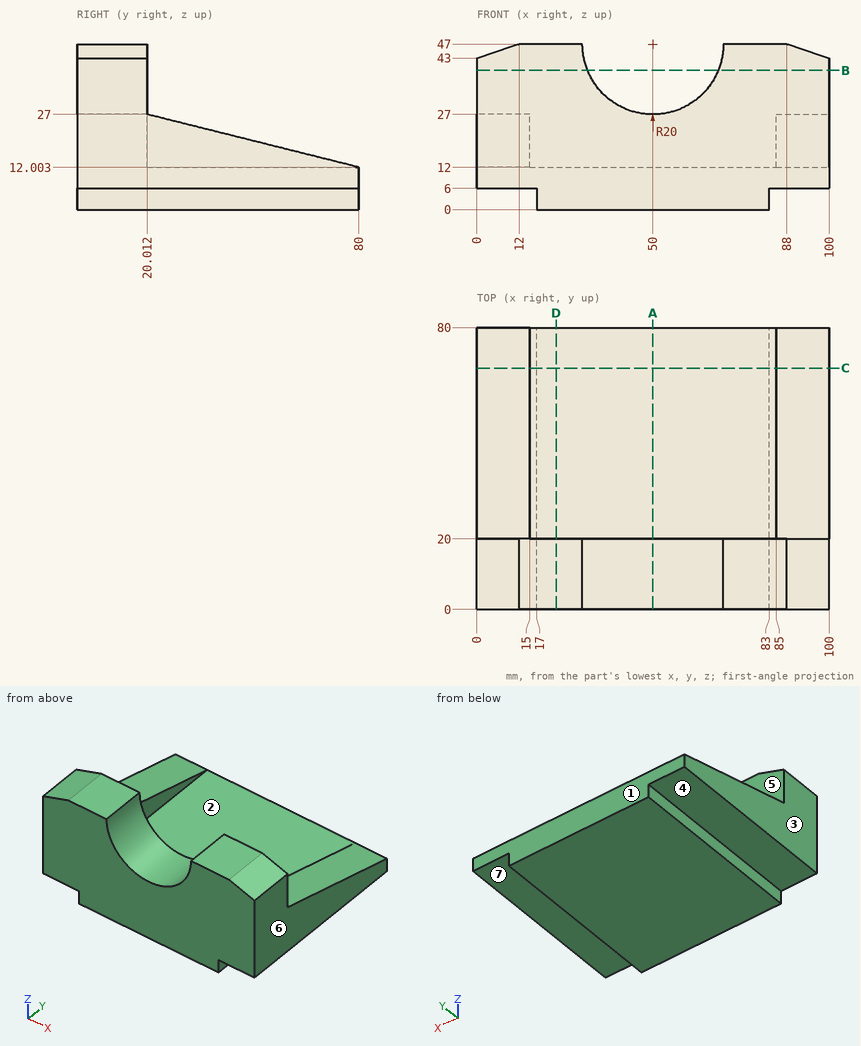
For this review, use the dimensioned drawing (mm, ordinates from the lowest corner) and the shaded views. A direction names the side the tool comes from. Give positions to 0.01 mm unless a question says otherwise; leave off trailing zeros. Write each loop counter-clockwise with the first axis right and the second up, starting at its lowest first coordinate (ties: lowest second). Pieces come first, ordered by that corner, then holes. Notation, with made-up numbers: M -8,60 L 12,60 A22 cw 12,78 Z; hole C 2,19 d9. An arc over 180 degrees is marked long. Answer as a JSON object with one key per item and string values. Group by question number.
1) We need section B-B (z = 39.5). Give the boundary of the cut face in (x, y).
2) Tool access review of the marked faces 4, 5, 6 and 7: name each direction out of +Z, -Z, +X, -X, +Y, -Y from which nothing blocks a thin tool from reaching the whole face with its end or side.
3) For line 1 along X through (y, z) = (41.5, 21); line 2 along Y through (x, z) = (34.5, 30); line 3 along Z through (x, y) = (41, 29), list the stretches that pass through material, from the lowest coordinate up.
4) We need section D-D (x = 22.5). Give the boundary of the cut face in (y, z), and give its area (3 significant figures).
5) Mouldability with a two-part tool opening along X and no side actions: class the marked faces 1, 2 and 3 as released by +X, released by -X, zero draft, split by the parting line, or undercut.
6) We need section A-A (x = 50). Give the boundary of the cut face in (y, z), and give its area (3 significant figures).
7) Clearance check with flat-ended pins moving along their axes: pin 1 Ø8 at (x, y) = (62.5, 57) entering from +Z; pin 2 Ø6.5 at (y, z) = (23, 2.5) entering from +X; pin 3 Ø1.8 at (y, z) = (58.5, 3) entering from -X. State where each tip first meets the part, or that it passes through.
8) We need section C-C (y = 68.5). Give the boundary of the cut face in (x, z), and give its area (3 significant figures).
Answer key:
{
 "1": {"outline": "M 0,0 L 31.46,0 L 31.46,20 L 0,20 Z; M 68.54,0 L 100,0 L 100,20 L 68.54,20 Z"},
 "2": {"face 4": "-Z, -X, +Y, -Y", "face 5": "+Z, +Y", "face 6": "+Z, -Z, +X, +Y, -Y", "face 7": "-Z, +X, +Y, -Y"},
 "3": {"line 1": "x = 0 to 15, 85 to 100", "line 2": "y = 0 to 20", "line 3": "z = 0 to 12"},
 "4": {"outline": "M 0,0 L 80,0 L 80,12 L 20,12 L 20,47 L 0,47 Z", "area": "1,660 mm²"},
 "5": {"face 1": "zero draft", "face 2": "undercut", "face 3": "released by -X"},
 "6": {"outline": "M 0,0 L 80,0 L 80,12 L 20,12 L 20,27 L 0,27 Z", "area": "1,260 mm²"},
 "7": {"pin 1": "stops at z = 12", "pin 2": "stops at x = 83", "pin 3": "stops at x = 17"},
 "8": {"outline": "M 0,6 L 17,6 L 17,0 L 83,0 L 83,6 L 100,6 L 100,14.88 L 85,14.88 L 85,12 L 15,12 L 15,14.88 L 0,14.88 Z", "area": "1,080 mm²"}
}
